Work out the finished part from the listing and answer in its coordinate system (mm). Face numbers are marked on the shaded views. Coordinates: 2 decimals unless noted, no trailing zeros. Write each loop counter-clockwise with the first axis right and the second up, starting at its lowest first coordinate (ties: lowest second). Pieces come first, ordered by that corner, then holes. Notation, with made-up numbers: (62, 54.5) - (77, 54.5) arc R27 cw to (77, 76.5) - close; hole circle Ø10 at (81, 22). An arc over 180 degrees is marked (long way). Use one line per item in the form item = value. Start each with the question number.
Item 1: A cutting plane is placed at A-A (x = 183). Write down the section's boundary in (y, z).
Item 2: Determine the mould class of the marked faces 1, 2 and 3 for opening direction Y: released by +Y, released by -Y, zero draft, split by the parting line, or undercut.
Item 3: Given pin 1 (6 mm diameter, centred on x = -56.5, z = 19, fed in from -Y); pin 2 (10.5 mm diameter, centred on x = 237, y = 54, fed in from +Z); pin 3 (6 mm diameter, centred on x = 125.5, y = 225, fed in from -Z), each flat-ended and moving along its own axis, determine where each tip first touches the part or whether it passes through.
Item 4: A cutting plane is placed at C-C (x = 0). Write down the section's boundary in (y, z), then the cut area to 3 significant figures.
Item 5: Consider probe 1 along Y at (x, z) = (0, 33.7); probe 2 along Y at (x, z) = (129, 48.55); probe 3 along X at (y, z) = (232, 101). Determine where each line is inside the solid, lowest interval first.
Item 6: A cutting plane is placed at D-D (z = 66.5). Write down the section's boundary in (x, y), then the cut area to 3 significant figures.
Item 7: A cutting plane is placed at B-B (y = -253). Write down the section's boundary in (x, z).
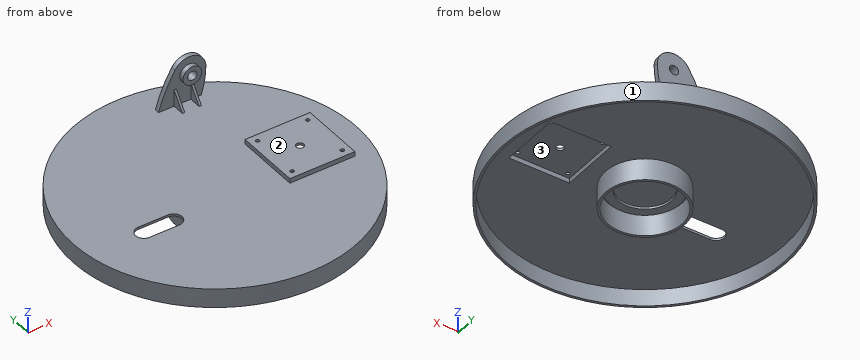
from build123d import *

# Parameters (mm, degrees)
SKETCH_1_R          = 305
EXTRUDE_1_DEPTH     = 41.2
SKETCH_2_W          = 140
SKETCH_2_H          = 140
EXTRUDE_2_DEPTH     = 10
SHELL_1_T           = -5
CUT_EXTRUDE_1_DEPTH = 10
SKETCH_4_W          = 120
SKETCH_4_H          = 10
EXTRUDE_3_DEPTH     = 150
CUT_EXTRUDE_2_DEPTH = 648.322516216
SKETCH_7_R          = 10
CUT_EXTRUDE_3_DEPTH = 150
EXTRUDE_START       = 10
SKETCH_8_R          = 20
SKETCH_8_R_2        = 10
EXTRUDE_4_DEPTH     = 10
SKETCH_9_W          = 5
SKETCH_9_H          = 36
EXTRUDE_5_DEPTH     = 26
CUT_EXTRUDE_4_DEPTH = 505.336286618
SKETCH_11_W         = 18
SKETCH_11_H         = 5
SKETCH_11_W_2       = 5
SKETCH_11_H_2       = 46.5
SKETCH_12_R         = 4
SKETCH_12_R_2       = 8
CUT_EXTRUDE_5_DEPTH = 26


with BuildPart() as part:
    # 草图1 → 凸台-拉伸1 (new body)
    with BuildSketch(Plane.XY):
        with Locations(Location((0, 0, 0), (0, 0, 180))):
            Circle(SKETCH_1_R)
    extrude(amount=EXTRUDE_1_DEPTH)

    # 草图2 → 凸台-拉伸2 (add)
    with BuildSketch(Plane.XY.offset(41.2)):
        with Locations((183, 0)):
            Rectangle(SKETCH_2_W, SKETCH_2_H)
    extrude(amount=EXTRUDE_2_DEPTH)

    # 抽壳1
    shell_1_openings = [part.faces().sort_by_distance(p)[0] for p in [
        (0, 0, 0),
    ]]
    offset(amount=SHELL_1_T, openings=shell_1_openings, kind=Kind.INTERSECTION)

    # 草图3 → 切除-拉伸1 (cut)
    with BuildSketch(Plane.XY.offset(41.2)):
        with BuildLine():
            Line((-182, -24), (-118, -24))
            ThreePointArc((-118, -24), (-100, -42), (-118, -60))
            Line((-118, -60), (-182, -60))
            ThreePointArc((-182, -60), (-200, -42), (-182, -24))
        make_face()
    extrude(amount=-CUT_EXTRUDE_1_DEPTH, mode=Mode.SUBTRACT)

    # 草图4 → 凸台-拉伸3 (add)
    with BuildSketch(Plane.XY.offset(41.2)):
        with Locations((99, 238)):
            Rectangle(SKETCH_4_W, SKETCH_4_H)
    extrude(amount=EXTRUDE_3_DEPTH)

    # 草图6 → 切除-拉伸2 (cut, through all)
    with BuildSketch(Plane.XZ.offset(-233)):
        with BuildLine():
            Line((39, 191.2), (39, 41.2))
            ThreePointArc((39, 41.2), (53.931588882, 82.177347592), (74.646786984, 120.556716136))
            ThreePointArc((74.646786984, 120.556716136), (115.26317996, 135.706044936), (140.99801314, 100.821780537))
            ThreePointArc((140.99801314, 100.821780537), (138.32356193, 70.621084147), (131, 41.2))
            Line((131, 41.2), (159, 41.2))
            Line((159, 41.2), (159, 191.2))
            Line((159, 191.2), (39, 191.2))
        make_face()
    extrude(amount=-CUT_EXTRUDE_2_DEPTH, mode=Mode.SUBTRACT)

    # 草图7 → 切除-拉伸3 (cut)
    with BuildSketch(Plane.XZ.offset(-233)):
        with Locations(Location((105, 101.2, 0), (0, 0, 270))):
            Circle(SKETCH_7_R)
    extrude(amount=-CUT_EXTRUDE_3_DEPTH, mode=Mode.SUBTRACT)

    # 草图8 → 凸台-拉伸4 (add)
    with BuildSketch(Plane.XZ.offset(-233).offset(EXTRUDE_START)):
        with Locations(Location((105, 101.2, 0), (0, 0, 90))):
            Circle(SKETCH_8_R)
        with Locations(Location((105, 101.2, 0), (0, 0, 270))):
            Circle(SKETCH_8_R_2, mode=Mode.SUBTRACT)
    extrude(amount=-EXTRUDE_4_DEPTH)

    # 草图9 → 凸台-拉伸5 (add)
    with BuildSketch(Plane.XZ.offset(-233)):
        with Locations((75, 59.2)):
            Rectangle(SKETCH_9_W, SKETCH_9_H)
        with Locations((111, 59.2)):
            Rectangle(SKETCH_9_W, SKETCH_9_H)
    extrude(amount=EXTRUDE_5_DEPTH)

    # 草图10 → 切除-拉伸4 (cut, through all)
    with BuildSketch(Plane.ZY.offset(-72.5)):
        Polygon((77.2, 233), (41.2, 207), (77.2, 207), align=None)
    extrude(amount=-CUT_EXTRUDE_4_DEPTH, mode=Mode.SUBTRACT)

    # 草图11 → 旋转1 (revolve)
    with BuildSketch(Plane(origin=(0, 0, 0), x_dir=(1, 0, 0), z_dir=(0, 1, 0)), mode=Mode.PRIVATE) as revolve_1_sk:
        with Locations((-66, -33.7)):
            Rectangle(SKETCH_11_W, SKETCH_11_H)
        with Locations((-82.5, -12.95)):
            Rectangle(SKETCH_11_W_2, SKETCH_11_H_2)
    revolve(revolve_1_sk.sketch.rotate(Axis((0, 0, 0), (0, 0, -1)), 180), axis=Axis((0, 0, 0), (0, 0, -1)))

    # 草图12 → 切除-拉伸5 (cut)
    with BuildSketch(Plane.XY.offset(51.2)):
        with Locations((237, 54)):
            Circle(SKETCH_12_R)
        with Locations((237, -54)):
            Circle(SKETCH_12_R)
        with Locations((129, -54)):
            Circle(SKETCH_12_R)
        with Locations((129, 54)):
            Circle(SKETCH_12_R)
        with Locations((183, 0)):
            Circle(SKETCH_12_R_2)
    extrude(amount=-CUT_EXTRUDE_5_DEPTH, mode=Mode.SUBTRACT)


solid = part.part
Answer:
q1.outline = (-244, 0) - (-237.72, 0) - (-237.72, 36.2) - (-65, 36.2) - (-65, 46.2) - (-8, 46.2) - (-8, 51.2) - (-70, 51.2) - (-70, 41.2) - (-244, 41.2) - close; (8, 46.2) - (65, 46.2) - (65, 36.2) - (237.72, 36.2) - (237.72, 0) - (244, 0) - (244, 41.2) - (70, 41.2) - (70, 51.2) - (8, 51.2) - close
q2.face_1 = split by the parting line
q2.face_2 = zero draft
q2.face_3 = undercut
q3.pin_1 = -300.27
q3.pin_2 = 51.2
q3.pin_3 = 36.2
q4.outline = (-305, 0) - (-300, 0) - (-300, 36.2) - (-85, 36.2) - (-85, -10.3) - (-80, -10.3) - (-80, 36.2) - (-75, 36.2) - (-75, 31.2) - (-57, 31.2) - (-57, 36.2) - (57, 36.2) - (57, 31.2) - (75, 31.2) - (75, 36.2) - (80, 36.2) - (80, -10.3) - (85, -10.3) - (85, 36.2) - (300, 36.2) - (300, 0) - (305, 0) - (305, 41.2) - (-305, 41.2) - close
q4.area = 4,060 mm²
q5.probe_1 = -305 to -300, -85 to -80, -75 to -57, 57 to 75, 80 to 85, 300 to 305
q5.probe_2 = -70 to -58, -50 to 50, 58 to 70, 233 to 243
q5.probe_3 = 85 to 95, 115 to 125
q6.outline = (47.42, 233) - (72.5, 233) - (72.5, 225.27) - (77.5, 225.27) - (77.5, 233) - (108.5, 233) - (108.5, 225.27) - (113.5, 225.27) - (113.5, 233) - (137.59, 233) - (137.59, 243) - (47.42, 243) - close
q6.area = 979 mm²
q7.outline = (-170.34, 0) - (-161.22, 0) - (-161.22, 36.2) - (161.22, 36.2) - (161.22, 0) - (170.34, 0) - (170.34, 41.2) - (-170.34, 41.2) - close
